The figure shows three views and two pictorial views of one solid part (mm, origin at its lowest corner). Answer the questions. Round coordinates to 2 decimals unless told otherwise and drop trailing zeros. Write each loop counter-clockwise with the first axis right and the second up, starting at its lowest first coordinate (ties: lowest second). Pieces come first, ordered by that corner, then holes.
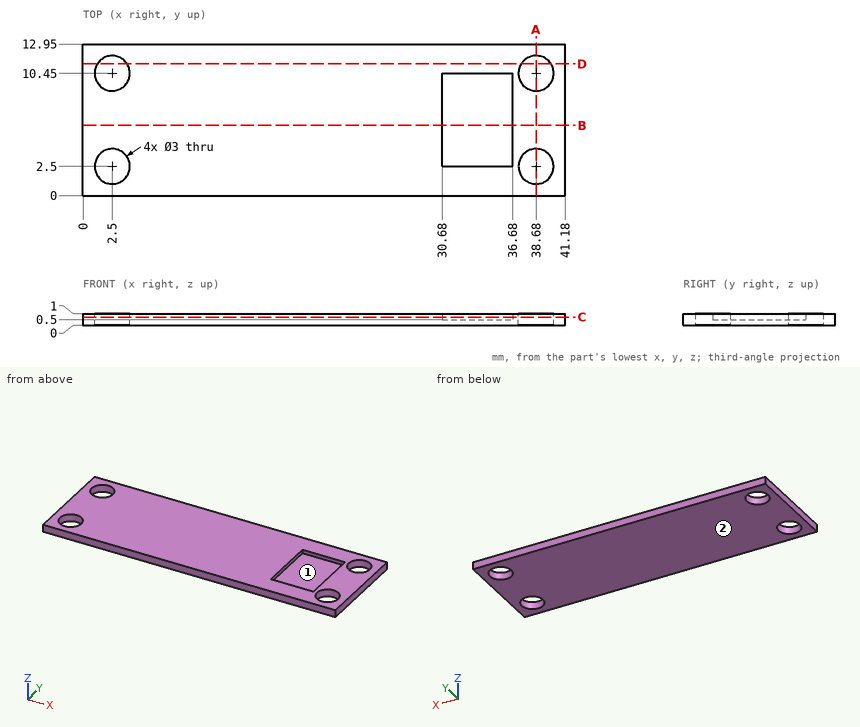
Q1. A flat-ended cylindrical pin translates along its axis: pin 1 Ø1.8 at (x, y) = (33, 6.5) entering from +Z. Find the tip coordinate at first contact, or state that the pin passes through.
Verdict:
pin 1: stops at z = 0.5
Q2. Section C-C (z = 0.7) is taken. Determine the outline of the cut face in (x, y), then the cut area to 3 significant figures.
Verdict:
outline: (0, 0) - (41.18, 0) - (41.18, 12.95) - (0, 12.95) - close; hole circle Ø3 at (2.5, 2.5); hole circle Ø3 at (2.5, 10.45); hole (30.68, 2.5) - (36.68, 2.5) - (36.68, 10.45) - (30.68, 10.45) - close; hole circle Ø3 at (38.68, 2.5); hole circle Ø3 at (38.68, 10.45)
area: 457 mm2
Q3. Section A-A (x = 38.68) is taken. Determine the outline of the cut face in (y, z).
Verdict:
outline: (0, 0) - (1, 0) - (1, 1) - (0, 1) - close; (4, 0) - (8.95, 0) - (8.95, 1) - (4, 1) - close; (11.95, 0) - (12.95, 0) - (12.95, 1) - (11.95, 1) - close
Q4. Straight lines are drawn through the part: probe 1 along Y at (x, z) = (38.68, 0.6); probe 2 along X at (y, z) = (6, 0.8); probe 3 along X at (y, z) = (2.25, 0.1). For each, find the intervals that lie inside material, in ascending order.
Verdict:
probe 1: y = 0 to 1, 4 to 8.95, 11.95 to 12.95
probe 2: x = 0 to 30.68, 36.68 to 41.18
probe 3: x = 0 to 1.02, 3.98 to 37.2, 40.16 to 41.18
Q5. Determine the mould class of the marked faces 1 and 2 for opening direction X: pulls with the +X half, pulls with the -X half, needs draft (parallel to the pull), parting line crosses it, or undercut.
Verdict:
face 1: undercut
face 2: needs draft
Q6. Section D-D (y = 11.25) is taken. Determine the outline of the cut face in (x, z), then the cut area to 3 significant figures.
Verdict:
outline: (0, 0) - (1.23, 0) - (1.23, 1) - (0, 1) - close; (3.77, 0) - (37.41, 0) - (37.41, 1) - (3.77, 1) - close; (39.95, 0) - (41.18, 0) - (41.18, 1) - (39.95, 1) - close
area: 36.1 mm2
Q7. Section B-B (y = 6) is taken. Determine the outline of the cut face in (x, z).
Verdict:
outline: (0, 0) - (41.18, 0) - (41.18, 1) - (36.68, 1) - (36.68, 0.5) - (30.68, 0.5) - (30.68, 1) - (0, 1) - close
